Answer from the drawing. Dimensions are ordinates in mm from the lowest x, y and z of the part. A direction names the side the tool comes from. Give positions to 0.01 mm unless a question says otherwise; leave off trailing zeros. Write each loop counter-clockwise with the first axis right and the second up, starting at its lowest first coordinate (ties: lowest second). Pieces come first, ordered by that corner, then holes. Notation, with made-up numbers: (-7.5, -26.5) - (27.5, -26.5) arc R30 cw to (27.5, -1.5) - close; hole circle Ø4 at (87, 89). An arc over 180 degrees is marked (long way). Write item = value, one per line.
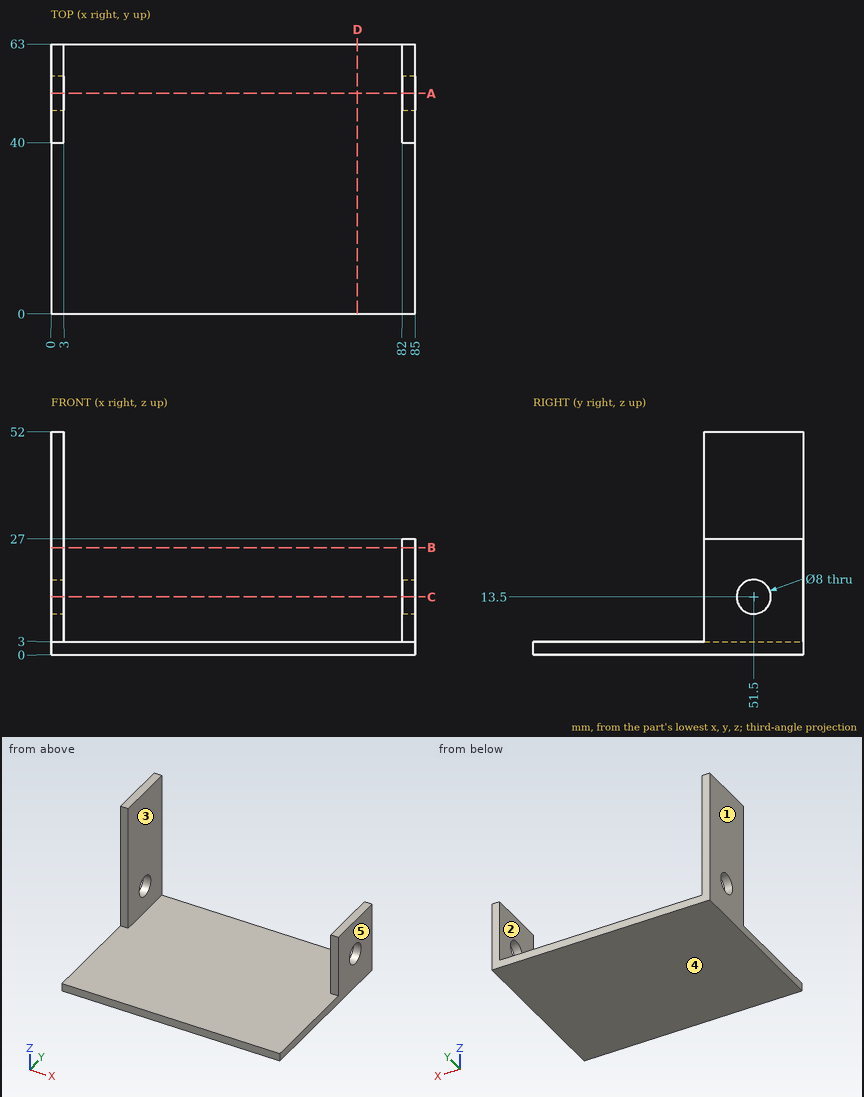
1. A tool of negligible diameter and unlimited length cuts with its end or side. For the marked faces 1 and 2, from which of +Z, -Z, +X, -X, +Y, -Y can it reach the whole face along a straight path? Write none if from no direction.
Solution:
face_1 = +Z, -Z, -X, +Y, -Y
face_2 = +Z, +Y, -Y
2. Find section C-C, the plane z = 13.5. Give the vertices of the cut face in (x, y).
Solution:
outline = (0, 40) - (3, 40) - (3, 47.5) - (0, 47.5) - close; (0, 55.5) - (3, 55.5) - (3, 63) - (0, 63) - close; (82, 40) - (85, 40) - (85, 47.5) - (82, 47.5) - close; (82, 55.5) - (85, 55.5) - (85, 63) - (82, 63) - close
3. Find section B-B, the plane z = 25. Give the vertices of the cut face in (x, y), then the cut area to 3 significant figures.
Solution:
outline = (0, 40) - (3, 40) - (3, 63) - (0, 63) - close; (82, 40) - (85, 40) - (85, 63) - (82, 63) - close
area = 138 mm^2
4. Find section A-A, the plane y = 51.5. Give the vertices of the cut face in (x, z).
Solution:
outline = (0, 0) - (85, 0) - (85, 9.5) - (82, 9.5) - (82, 3) - (3, 3) - (3, 9.5) - (0, 9.5) - close; (0, 17.5) - (3, 17.5) - (3, 52) - (0, 52) - close; (82, 17.5) - (85, 17.5) - (85, 27) - (82, 27) - close
5. For a pull along X with two mould halves and no side action, classify the marked faces 3, 4 and 5 as pulls with the +X half, pulls with the -X half, needs draft (parallel to the pull), parting line crosses it, or undercut.
Solution:
face_3 = undercut
face_4 = needs draft
face_5 = pulls with the +X half
6. Straight lines are drawn through the part: line 1 (X direction, y = 57, z = 10.5); line 2 (Z direction, x = 82.7, y = 51.5); line 3 (Z direction, x = 2, y = 51.5). For each, find the intervals that lie inside material, in ascending order.
Solution:
line_1 = 0 to 3, 82 to 85
line_2 = 0 to 9.5, 17.5 to 27
line_3 = 0 to 9.5, 17.5 to 52
7. Given pin 1 (7 mm diameter, centred on y = 57, z = 38.5, fed in from +X); pin 2 (8 mm diameter, centred on y = 32.5, z = 18, fed in from -X); pin 3 (1.5 mm diameter, centred on x = 83, y = 48.5, fed in from +Z); pin 4 (1.5 mm diameter, centred on x = 84, z = 17, fed in from -Y), each flat-ended and moving along its own axis, determine where each tip first touches the part or whether it passes through.
Solution:
pin_1 = 3
pin_2 = through
pin_3 = 27
pin_4 = 40
8. Find section D-D, the plane x = 71.5. Give the vertices of the cut face in (y, z), then the cut area to 3 significant figures.
Solution:
outline = (0, 0) - (63, 0) - (63, 3) - (0, 3) - close
area = 189 mm^2
